Source: CAD feature listing. Evaluate the final solid. Frame: model axes, mm. Face numbers are marked on the shaded views. A direction names the side the tool comes from. Round coordinates to 2 decimals unless told otherwise and drop trailing zeros. Order: outer loops, then holes, each group sorted by start corner. A loop starts at its lowest first (then second) coordinate and runs counter-clockwise, first axis right, second up. Notation, with made-up numbers: M 30,83 L 35,83 A23 ccw 35,102 Z; hole C 38.25,44 d3. An arc over 180 degrees is marked long. Use one line per item in the form item = value. Start each with the question number.
Q1. Section C-C (x = 2.8). Return the cut outline in (y, z).
Q2. Section B-B (y = 7.25). Return the cut outline in (x, z).
Q3. Reachability of the marked faces 1, 2, 3 and 4 from +Z, -Z, +X, -X, +Y, -Y: full face, straight path, thin tool, end or side. Return the list, or none.
Q4. Section A-A (y = -4.5). Return the cut outline in (x, z), plus the area to 3 significant figures.
Q5. Contact query for flat-ended pins moving along their axis: pin 1 (1.6 mm diameter, centred on x = 2, z = -32.5, fed in from -Y); pin 2 (3 mm diameter, centred on x = 2, z = -26, fed in from +Y); pin 3 (3 mm diameter, centred on x = 3, y = -10.5, fed in from +Z); pin 4 (3 mm diameter, centred on x = 3, y = -3.5, fed in from -Z). Output: stop coordinate, or through.
Q6. Material intervals for probe 1 along Z at (x, y) = (4.65, -7.5); probe 2 along Z at (x, y) = (3.1, 11); probe 3 along Z at (x, y) = (4.1, 7), sorted ascending.
Q7. Section D-D (z = -3). Return the cut outline in (x, y).
Autodesk Inventor part; units mm, degrees
ref_plane "YZ Plane" through (0, 0, 0) normal (1, 0, 0) x (0, 1, 0)
ref_plane "XZ Plane" through (0, 0, 0) normal (0, 1, 0) x (-1, 0, 0)
ref_plane "XY Plane" through (0, 0, 0) normal (0, 0, 1) x (1, 0, 0)
sketch "Esquisse1" plane through (0, 0, 0) normal (1, 0, 0) x (0, 1, 0)
  line L0 (-5.5, 0) -> (5.5, 0)
  line L1 (10.5, -8) -> (4, -8)
  line L2 (4, -8) -> (4, -13)
  line L3 (4, -13) -> (14, -13)
  line L4 (14, -13) -> (14, -18)
  line L5 (14, -18) -> (4, -18)
  line L6 (-10.5, -8) -> (-4, -8)
  line L7 (-4, -8) -> (-4, -13)
  line L8 (-4, -13) -> (-14, -13)
  line L9 (-14, -13) -> (-14, -18)
  line L10 (-14, -18) -> (-4, -18)
  line L11 (4, -18) -> (4, -33)
  line L12 (-4, -18) -> (-4, -41)
  line L13 (5.5, 0) -> (10.5, -5)
  line L14 (10.5, -5) -> (10.5, -8)
  line L15 (-5.5, 0) -> (-10.5, -5)
  line L16 (-10.5, -5) -> (-10.5, -8)
  line L17 (14, -33) -> (14, -41)
  line L18 (4, -33) -> (14, -33)
  line L19 (14, -41) -> (-4, -41)
  point P0 (0, 0)
  point P1 (0, 0)
  dimension "d0" = 8
  dimension "d1" = 8
  dimension "d2" = 3
  dimension "d3" = 10
  dimension "d6" = 5
  dimension "d7" = 5
  dimension "d10" = 21
  dimension "d11" = 45
  dimension "d14" = 10
  dimension "d15" = 8
  dimension "d16" = 15
  dimension "d17" = 28
  dimension "d18" = 28
extrude "Extrusion1" add sketch "Esquisse1" along normal blind 5.5
fillet "Congé1" radius 2 2 edges at (2.75, -4, -41) (2.75, 4, -33)
properties part number "cable holder"
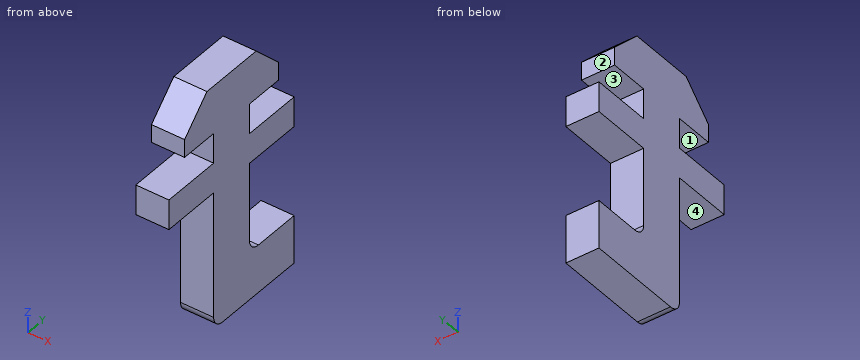
Results list:
q1.outline = M -14,-18 L -4,-18 L -4,-39 A2 ccw -2,-41 L 14,-41 L 14,-33 L 6,-33 A2 cw 4,-31 L 4,-18 L 14,-18 L 14,-13 L 4,-13 L 4,-8 L 10.5,-8 L 10.5,-5 L 5.5,0 L -5.5,0 L -10.5,-5 L -10.5,-8 L -4,-8 L -4,-13 L -14,-13 Z
q2.outline = M 0,-41 L 5.5,-41 L 5.5,-33 L 0,-33 Z; M 0,-18 L 5.5,-18 L 5.5,-13 L 0,-13 Z; M 0,-8 L 5.5,-8 L 5.5,-1.75 L 0,-1.75 Z
q3.face_1 = +X, -X, -Y
q3.face_2 = +Z, +X, -X, +Y
q3.face_3 = +X, -X, +Y
q3.face_4 = -Z, +X, -X, -Y
q4.outline = M 0,-18 L 5.5,-18 L 5.5,-13 L 0,-13 Z; M 0,-8 L 5.5,-8 L 5.5,0 L 0,0 Z
q4.area = 71.5 mm2
q5.pin_1 = -4
q5.pin_2 = 4
q5.pin_3 = -3.5
q5.pin_4 = -41
q6.probe_1 = -18 to -13, -8 to -2
q6.probe_2 = -41 to -33, -18 to -13
q6.probe_3 = -41 to -33, -18 to -13, -8 to -1.5
q7.outline = M 0,-8.5 L 5.5,-8.5 L 5.5,8.5 L 0,8.5 Z
